Can you work these out from the model? Positions are in its coordinate system, mm. Coordinates: 2 decimals unless noted, no trailing zeros. Order: outer loops, then holes, each group sorted by start corner. A loop starts at its lowest first (then second) coordinate and runs counter-clockwise, first axis right, second up. Notation, with made-up numbers: (10, -1) -> (52, -1) arc R25 ccw to (52, 21) -> close; hole circle Ø2 at (89, 74). An arc over 180 degrees is marked (long way). Use a Markdown table: item, result. Add a question column.
1. Suppose I cut it at C-C, the plane x = 18. List the corners of the cut face in (y, z) for me, then the cut area to 3 significant figures.
2. If I drill on line 1 along X through (y, z) = (0.7, 24.5); line 2 along Z through (x, y) = (23.57, 2.05); line 3 along Z through (x, y) = (-24, 0.85), over which ranges is the centre line in solid material (lowest first)? Write a range as from..to.
3. Suppose I cut it at D-D, the plane z = 23.57. List the corners of the cut face in (x, y) for me.
4. Suppose I cut it at A-A, the plane z = 0. List the corners of the cut face in (x, y) for me, then the cut area to 3 significant figures.
5. Suppose I cut it at B-B, the plane x = 0. List the corners of the cut face in (y, z) for me, then the cut area to 3 significant figures.
6. For pin 1 Ø1.6 at (x, y) = (-32, 3) entering from -Z; pin 2 Ø1.2 at (x, y) = (-39, 2) entering from +Z; pin 3 Ø2.5 at (x, z) = (23.57, -23.57) entering from +Y; pin 4 Ø2 at (x, y) = (-1, 2.5) entering from -Z, each with a flat end and sliding along its axis, tell me the tip position at first contact or that it passes through.
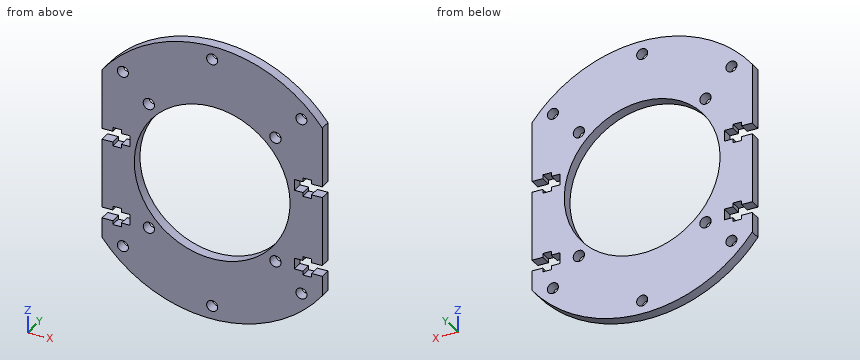
```python
from build123d import *

# Parameters (mm, degrees)
SKETCH_1_R          = 52
SKETCH_1_R_2        = 29
SKETCH_1_R_3        = 2.05
SKETCH_1_R_4        = 2.1
EXTRUDE_1_DEPTH     = 4
SKETCH_2_W          = 182
SKETCH_2_H          = 210.035227354
SKETCH_2_W_2        = 82
SKETCH_2_H_2        = 110.035227354
CUT_EXTRUDE_1_DEPTH = 4


with BuildPart() as part:
    # 草图1 → 凸台-拉伸1 (new body)
    with BuildSketch(Plane(origin=(0, 0, 0), x_dir=(1, 0, 0), z_dir=(0, 1, 0))):
        with Locations(Location((0, 0, 0), (0, 0, 270))):
            Circle(SKETCH_1_R)
        with Locations(Location((0, 0, 0), (0, 0, 270))):
            Circle(SKETCH_1_R_2, mode=Mode.SUBTRACT)
        with Locations(Location((47, 0, 0), (0, 0, 270))):
            Circle(SKETCH_1_R_3, mode=Mode.SUBTRACT)
        with Locations(Location((33.234018716, -33.234018716, 0), (0, 0, 270))):
            Circle(SKETCH_1_R_3, mode=Mode.SUBTRACT)
        with Locations(Location((0, -47, 0), (0, 0, 270))):
            Circle(SKETCH_1_R_3, mode=Mode.SUBTRACT)
        with Locations(Location((-33.234018716, -33.234018716, 0), (0, 0, 270))):
            Circle(SKETCH_1_R_3, mode=Mode.SUBTRACT)
        with Locations(Location((-47, 0, 0), (0, 0, 270))):
            Circle(SKETCH_1_R_3, mode=Mode.SUBTRACT)
        with Locations(Location((-33.234018716, 33.234018716, 0), (0, 0, 270))):
            Circle(SKETCH_1_R_3, mode=Mode.SUBTRACT)
        with Locations(Location((0, 47, 0), (0, 0, 270))):
            Circle(SKETCH_1_R_3, mode=Mode.SUBTRACT)
        with Locations(Location((33.234018716, 33.234018716, 0), (0, 0, 270))):
            Circle(SKETCH_1_R_3, mode=Mode.SUBTRACT)
        with Locations(Location((-23.57, 23.57, 0), (0, 0, 270))):
            Circle(SKETCH_1_R_4, mode=Mode.SUBTRACT)
        with Locations(Location((-23.57, -23.57, 0), (0, 0, 270))):
            Circle(SKETCH_1_R_4, mode=Mode.SUBTRACT)
        with Locations(Location((23.57, -23.57, 0), (0, 0, 90))):
            Circle(SKETCH_1_R_4, mode=Mode.SUBTRACT)
        with Locations(Location((23.57, 23.57, 0), (0, 0, 90))):
            Circle(SKETCH_1_R_4, mode=Mode.SUBTRACT)
        Polygon((37, -9.55), (37, -11), (33.8, -11), (33.8, -9.55), (30.6, -9.55), (30.6, -5.45), (33.8, -5.45), (33.8, -4), (37, -4), (37, -5.45), (41, -5.45), (41, -9.55), align=None, mode=Mode.SUBTRACT)
        Polygon((37, 20.45), (37, 19), (33.8, 19), (33.8, 20.45), (30.6, 20.45), (30.6, 24.55), (33.8, 24.55), (33.8, 26), (37, 26), (37, 24.55), (41, 24.55), (41, 20.45), align=None, mode=Mode.SUBTRACT)
        Polygon((-33.8, 26), (-37, 26), (-37, 24.55), (-41, 24.55), (-41, 20.45), (-37, 20.45), (-37, 19), (-33.8, 19), (-33.8, 20.45), (-30.6, 20.45), (-30.6, 24.55), (-33.8, 24.55), align=None, mode=Mode.SUBTRACT)
        Polygon((-33.8, -4), (-37, -4), (-37, -5.45), (-41, -5.45), (-41, -9.55), (-37, -9.55), (-37, -11), (-33.8, -11), (-33.8, -9.55), (-30.6, -9.55), (-30.6, -5.45), (-33.8, -5.45), align=None, mode=Mode.SUBTRACT)
    extrude(amount=EXTRUDE_1_DEPTH)

    # 草图2 → 切除-拉伸-薄壁1 (cut)
    with BuildSketch(Plane(origin=(0, 4, 0), x_dir=(1, 0, 0), z_dir=(0, 1, 0))):
        Rectangle(SKETCH_2_W, SKETCH_2_H)
        Rectangle(SKETCH_2_W_2, SKETCH_2_H_2, mode=Mode.SUBTRACT)
    extrude(amount=-CUT_EXTRUDE_1_DEPTH, mode=Mode.SUBTRACT)


solid = part.part
```
Worked out:
| question | item | result |
|---|---|---|
| 1 | outline | (0, -48.79) -> (4, -48.79) -> (4, -22.74) -> (0, -22.74) -> close; (0, 22.74) -> (4, 22.74) -> (4, 48.79) -> (0, 48.79) -> close |
| 1 | area | 208 mm² |
| 2 | line 1 | x = -41..-25.45, -21.69..-15.52, 15.52..21.69, 25.45..41 |
| 2 | line 2 | z = -46.35..-25.67, -21.47..-16.9, 16.9..21.47, 25.67..46.35 |
| 2 | line 3 | z = -46.13..-25.63, -21.51..-16.28, 16.28..21.51, 25.63..46.13 |
| 3 | outline | (-41, 0) -> (-25.67, 0) -> (-25.67, 4) -> (-41, 4) -> close; (-21.47, 0) -> (-16.9, 0) -> (-16.9, 4) -> (-21.47, 4) -> close; (16.9, 0) -> (21.47, 0) -> (21.47, 4) -> (16.9, 4) -> close; (25.67, 0) -> (41, 0) -> (41, 4) -> (25.67, 4) -> close |
| 4 | outline | (-41, 0) -> (-29, 0) -> (-29, 4) -> (-41, 4) -> close; (29, 0) -> (41, 0) -> (41, 4) -> (29, 4) -> close |
| 4 | area | 96.0 mm² |
| 5 | outline | (0, -52) -> (4, -52) -> (4, -49.05) -> (0, -49.05) -> close; (0, -44.95) -> (4, -44.95) -> (4, -29) -> (0, -29) -> close; (0, 29) -> (4, 29) -> (4, 44.95) -> (0, 44.95) -> close; (0, 49.05) -> (4, 49.05) -> (4, 52) -> (0, 52) -> close |
| 5 | area | 151 mm² |
| 6 | pin 1 | stops at z = -41.6 |
| 6 | pin 2 | stops at z = 35.06 |
| 6 | pin 3 | passes through |
| 6 | pin 4 | stops at z = -52 |
